```python
from build123d import *

# Parameters (mm, degrees)
SKETCH_1_R           = 20.68
SKETCH_1_R_2         = 9.68
EXTRUDE_1_DEPTH      = 116.68
SKETCH_11_W          = 27
SKETCH_11_H          = 150
CUT_EXTRUDE_3_DEPTH  = 40
SKETCH_13_W          = 10
SKETCH_13_H          = 128.345013401
CUT_EXTRUDE_7_DEPTH  = 126.614916312
SKETCH_15_W          = 8
SKETCH_15_H          = 68.68
CUT_EXTRUDE_9_DEPTH  = 48
SKETCH_16_W          = 15.549431524
SKETCH_16_H          = 20
SKETCH_16_W_2        = 15.459431524
EXTRUDE_4_DEPTH      = 19.2
SKETCH_17_W          = 19.20851187
SKETCH_17_H          = 14.03
CUT_EXTRUDE_10_DEPTH = 20.2
SKETCH_18_R          = 9.59
CUT_EXTRUDE_11_DEPTH = 121.289430957
SKETCH_21_R          = 2.985
CUT_EXTRUDE_12_DEPTH = 55.2
EXTRUDE_START        = 55.2
SKETCH_24_R          = 20.59
SKETCH_24_R_2        = 9.59
EXTRUDE_2_DEPTH      = 55.2
CUT_EXTRUDE_13_DEPTH = 55.2
SKETCH_26_W          = 10.00851187
SKETCH_26_H          = 41.68
CUT_EXTRUDE_15_DEPTH = 55.2
SKETCH_27_W          = 10
SKETCH_27_H          = 40
CUT_EXTRUDE_16_DEPTH = 55.2
SKETCH_28_W          = 44.880694938
SKETCH_28_H          = 9.608044066
CUT_EXTRUDE_17_DEPTH = 12.2
SKETCH_35_W          = 13.53
SKETCH_35_H          = 20
EXTRUDE_10_DEPTH     = 15
EXTRUDE_11_DEPTH     = 15
SKETCH_37_W          = 9
SKETCH_37_H          = 20
EXTRUDE_12_DEPTH     = 20
SKETCH_38_W          = 9
SKETCH_38_H          = 20
EXTRUDE_13_DEPTH     = 20
SKETCH_42_R          = 2.985
CUT_EXTRUDE_21_DEPTH = 20
CUT_EXTRUDE_23_DEPTH = 138.235841092
SKETCH_45_W          = 3
SKETCH_45_H          = 20
EXTRUDE_14_DEPTH     = 30
SKETCH_46_W          = 3
SKETCH_46_H          = 20
EXTRUDE_15_DEPTH     = 30
SKETCH_47_W          = 33.078221107
SKETCH_47_H          = 20
EXTRUDE_16_DEPTH     = 50
SKETCH_48_W          = 30
SKETCH_48_H          = 20
EXTRUDE_17_DEPTH     = 50
SKETCH_50_W          = 50
SKETCH_50_H          = 20
EXTRUDE_18_DEPTH     = 1
SKETCH_51_W          = 50
SKETCH_51_H          = 20
EXTRUDE_19_DEPTH     = 1
SKETCH_52_W          = 53
SKETCH_52_H          = 14
CUT_EXTRUDE_24_DEPTH = 151.972575738
SKETCH_53_W          = 53
SKETCH_53_H          = 14
CUT_EXTRUDE_25_DEPTH = 151.942387436
SKETCH_54_W          = 40
SKETCH_54_H          = 73.27
CUT_EXTRUDE_26_DEPTH = 147.866192927
SKETCH_56_W          = 13.00851187
SKETCH_56_H          = 20
EXTRUDE_21_DEPTH     = 3.08
SKETCH_57_R          = 2.985
CUT_EXTRUDE_27_DEPTH = 127.558817396


with BuildPart() as part:
    # 草圖1 → 伸長-薄件1 (new body)
    with BuildSketch(Plane(origin=(0, 0, 0), x_dir=(1, 0, 0), z_dir=(0, 1, 0))):
        Circle(SKETCH_1_R)
        Circle(SKETCH_1_R_2, mode=Mode.SUBTRACT)
    extrude(amount=EXTRUDE_1_DEPTH)

    # 草圖11 → 除料-伸長3 (cut)
    with BuildSketch(Plane(origin=(0, 116.68, 0), x_dir=(1, 0, 0), z_dir=(0, 1, 0))):
        with Locations((21.70851187, -44.235815192)):
            Rectangle(SKETCH_11_W, SKETCH_11_H)
    extrude(amount=-CUT_EXTRUDE_3_DEPTH, mode=Mode.SUBTRACT)

    # 草圖13 → 除料-伸長7 (cut, through all)
    with BuildSketch(Plane.XY.offset(21)):
        with Locations((-16, 58.612182466)):
            Rectangle(SKETCH_13_W, SKETCH_13_H)
    extrude(amount=-CUT_EXTRUDE_7_DEPTH, mode=Mode.SUBTRACT)

    # 草圖15 → 除料-伸長9 (cut)
    with BuildSketch(Plane.XY.offset(21)):
        with Locations((-1.395744065, 52.34)):
            Rectangle(SKETCH_15_W, SKETCH_15_H)
    extrude(amount=-CUT_EXTRUDE_9_DEPTH, mode=Mode.SUBTRACT)

    # 草圖16 → 填料-伸長4 (add)
    with BuildSketch(Plane(origin=(8.20851187, 0, 0), x_dir=(0, 0, -1), z_dir=(1, 0, 0))):
        with Locations((12.905284238, 106.68)):
            Rectangle(SKETCH_16_W, SKETCH_16_H)
        with Locations((-12.860284238, 106.68)):
            Rectangle(SKETCH_16_W_2, SKETCH_16_H)
    extrude(amount=-EXTRUDE_4_DEPTH)

    # 草圖17 → 除料-伸長10 (cut)
    with BuildSketch(Plane(origin=(0, 116.68, 0), x_dir=(1, 0, 0), z_dir=(0, 1, 0))):
        with Locations((-1.395744065, -0.045)):
            Rectangle(SKETCH_17_W, SKETCH_17_H)
    extrude(amount=-CUT_EXTRUDE_10_DEPTH, mode=Mode.SUBTRACT)

    # 草圖18 → 除料-伸長11 (cut, through all)
    with BuildSketch(Plane.XZ):
        with Locations(Location((0, 0, 0), (0, 0, 90))):
            Circle(SKETCH_18_R)
    extrude(amount=-CUT_EXTRUDE_11_DEPTH, mode=Mode.SUBTRACT)

    # 草圖21 → 除料-伸長12 (cut)
    with BuildSketch(Plane(origin=(0, 0, -20.68), x_dir=(-1, 0, 0), z_dir=(0, 0, -1))):
        with Locations((1.39148813, 108.73)):
            Circle(SKETCH_21_R)
    extrude(amount=-CUT_EXTRUDE_12_DEPTH, mode=Mode.SUBTRACT)

    # 草圖24 → 伸長-薄件2 (add)
    with BuildSketch(Plane.XZ.offset(EXTRUDE_START)):
        Circle(SKETCH_24_R)
        Circle(SKETCH_24_R_2, mode=Mode.SUBTRACT)
    extrude(amount=-EXTRUDE_2_DEPTH)

    # 草圖25 → 除料-伸長13 (cut)
    with BuildSketch(Plane.XY.offset(21)):
        Polygon((-1.39148813, -11.785), (22.612379708, -11.785), (22.612379708, -63.873337429), (-22.749525245, -63.873337429), (-22.749525245, -11.785), align=None)
    extrude(amount=-CUT_EXTRUDE_13_DEPTH, mode=Mode.SUBTRACT)

    # 草圖26 → 除料-伸長15 (cut)
    with BuildSketch(Plane(origin=(0, 0, 0), x_dir=(1, 0, 0), z_dir=(0, 1, 0))):
        with Locations((-15.995744065, -0.16)):
            Rectangle(SKETCH_26_W, SKETCH_26_H)
    extrude(amount=-CUT_EXTRUDE_15_DEPTH, mode=Mode.SUBTRACT)

    # 草圖27 → 除料-伸長16 (cut)
    with BuildSketch(Plane(origin=(21, 0, 0), x_dir=(0, 0, -1), z_dir=(1, 0, 0))):
        with Locations((0, 41.68)):
            Rectangle(SKETCH_27_W, SKETCH_27_H)
    extrude(amount=-CUT_EXTRUDE_16_DEPTH, mode=Mode.SUBTRACT)

    # 草圖28 → 除料-伸長17 (cut)
    with BuildSketch(Plane(origin=(21, 0, 0), x_dir=(0, 0, -1), z_dir=(1, 0, 0))):
        Rectangle(SKETCH_28_W, SKETCH_28_H)
    extrude(amount=-CUT_EXTRUDE_17_DEPTH, mode=Mode.SUBTRACT)

    # 草圖35 → 填料-伸長10 (add)
    with BuildSketch(Plane.ZY.offset(10.99148813)):
        with Locations((13.825, 106.68)):
            Rectangle(SKETCH_35_W, SKETCH_35_H)
    extrude(amount=EXTRUDE_10_DEPTH)

    # 草圖36 → 填料-伸長11 (add)
    with BuildSketch(Plane.ZY.offset(10.99148813)):
        Polygon((-20.68, 116.68), (-6.97, 116.68), (-6.97, 96.48), (-20.68, 96.68), align=None)
    extrude(amount=EXTRUDE_11_DEPTH)

    # 草圖37 → 填料-伸長12 (add)
    with BuildSketch(Plane.XY.offset(20.59)):
        with Locations((-21.49148813, 106.68)):
            Rectangle(SKETCH_37_W, SKETCH_37_H)
    extrude(amount=EXTRUDE_12_DEPTH)

    # 草圖38 → 填料-伸長13 (add)
    with BuildSketch(Plane(origin=(0, 0, -20.68), x_dir=(-1, 0, 0), z_dir=(0, 0, -1))):
        with Locations((21.49148813, 106.68)):
            Rectangle(SKETCH_38_W, SKETCH_38_H)
    extrude(amount=EXTRUDE_13_DEPTH)

    # 草圖42 → 除料-伸長21 (cut)
    with BuildSketch(Plane(origin=(-16.99148813, 0, 0), x_dir=(0, 0, -1), z_dir=(1, 0, 0))):
        with Locations((30.68, 106.554418142)):
            Circle(SKETCH_42_R)
        with Locations((-30.395640125, 106.68)):
            Circle(SKETCH_42_R)
    extrude(amount=-CUT_EXTRUDE_21_DEPTH, mode=Mode.SUBTRACT)

    # 草圖43 → 除料-伸長23 (cut, through all)
    with BuildSketch(Plane(origin=(0, 116.68, 0), x_dir=(1, 0, 0), z_dir=(0, 1, 0))):
        Polygon((-11, 6.97), (-10.99148813, 20.68), (-10.99148813, 48.096794253), (-28.274756234, 48.096794253), (-28.274756234, -43.270506289), (-11, -43.270506289), align=None)
    extrude(amount=-CUT_EXTRUDE_23_DEPTH, mode=Mode.SUBTRACT)

    # 草圖45 → 填料-伸長14 (add)
    with BuildSketch(Plane.XY.offset(20.59)):
        with Locations((-9.5, 106.68)):
            Rectangle(SKETCH_45_W, SKETCH_45_H)
    extrude(amount=EXTRUDE_14_DEPTH)

    # 草圖46 → 填料-伸長15 (add)
    with BuildSketch(Plane(origin=(0, 0, -20.68), x_dir=(-1, 0, 0), z_dir=(0, 0, -1))):
        with Locations((9.49148813, 106.68)):
            Rectangle(SKETCH_46_W, SKETCH_46_H)
    extrude(amount=EXTRUDE_15_DEPTH)

    # 草圖47 → 填料-伸長16 (add)
    with BuildSketch(Plane.ZY.offset(11)):
        with Locations((34.050889447, 106.68)):
            Rectangle(SKETCH_47_W, SKETCH_47_H)
    extrude(amount=EXTRUDE_16_DEPTH)

    # 草圖48 → 填料-伸長17 (add)
    with BuildSketch(Plane.ZY.offset(10.99148813)):
        with Locations((-35.68, 106.68)):
            Rectangle(SKETCH_48_W, SKETCH_48_H)
    extrude(amount=EXTRUDE_17_DEPTH)

    # 草圖50 → 填料-伸長18 (add)
    with BuildSketch(Plane(origin=(0, 0, 17.511778893), x_dir=(-1, 0, 0), z_dir=(0, 0, -1))):
        with Locations((36, 106.68)):
            Rectangle(SKETCH_50_W, SKETCH_50_H)
    extrude(amount=EXTRUDE_18_DEPTH)

    # 草圖51 → 填料-伸長19 (add)
    with BuildSketch(Plane.XY.offset(-20.68)):
        with Locations((-35.99148813, 106.68)):
            Rectangle(SKETCH_51_W, SKETCH_51_H)
    extrude(amount=EXTRUDE_19_DEPTH)

    # 草圖52 → 除料-伸長24 (cut, through all)
    with BuildSketch(Plane(origin=(0, 116.68, 0), x_dir=(1, 0, 0), z_dir=(0, 1, 0))):
        with Locations((-34.49148813, 43.68)):
            Rectangle(SKETCH_52_W, SKETCH_52_H)
    extrude(amount=-CUT_EXTRUDE_24_DEPTH, mode=Mode.SUBTRACT)

    # 草圖53 → 除料-伸長25 (cut, through all)
    with BuildSketch(Plane(origin=(0, 116.68, 0), x_dir=(1, 0, 0), z_dir=(0, 1, 0))):
        with Locations((-34.5, -43.59)):
            Rectangle(SKETCH_53_W, SKETCH_53_H)
    extrude(amount=-CUT_EXTRUDE_25_DEPTH, mode=Mode.SUBTRACT)

    # 草圖54 → 除料-伸長26 (cut, through all)
    with BuildSketch(Plane(origin=(0, 116.68, 0), x_dir=(1, 0, 0), z_dir=(0, 1, 0))):
        with Locations((-41, 0.045)):
            Rectangle(SKETCH_54_W, SKETCH_54_H)
    extrude(amount=-CUT_EXTRUDE_26_DEPTH, mode=Mode.SUBTRACT)

    # 草圖56 → 填料-伸長21 (add)
    with BuildSketch(Plane(origin=(0, 0, -36.68), x_dir=(-1, 0, 0), z_dir=(0, 0, -1))):
        with Locations((14.495744065, 106.68)):
            Rectangle(SKETCH_56_W, SKETCH_56_H)
    extrude(amount=EXTRUDE_21_DEPTH)

    # 草圖57 → 除料-伸長27 (cut, through all)
    with BuildSketch(Plane(origin=(-7.99148813, 0, 0), x_dir=(0, 0, -1), z_dir=(1, 0, 0))):
        with Locations((30.22, 106.634392252)):
            Circle(SKETCH_57_R)
        with Locations((-28.59, 106.68)):
            Circle(SKETCH_57_R)
    extrude(amount=-CUT_EXTRUDE_27_DEPTH, mode=Mode.SUBTRACT)


solid = part.part
```
Geometry check sheet. Reference: the model listing, model coordinates, mm. A direction names the side the tool comes from. Coordinates: 2 decimals unless noted, no trailing zeros. Loops run counter-clockwise (first coordinate to the right, second up) from the corner with the lowest first, then second, coordinate; pieces in that order, holes last. Notation, with made-up numbers: (28.25, -28.5) - (82.25, -28.5) arc R24 ccw to (82.25, 0.5) - close; hole circle Ø10 at (-3, -8). An arc over 180 degrees is marked (long way). One line per item, written item: value. Start each with the question number.
(1) Depth check by flat-ended pin: P1, Ø6, axis at x = -7, y = 71.5, coming from the -Z side; P2, Ø6, axis at y = 37.5, z = -14, coming from the +X side; P3, Ø2, axis at y = 9.5, z = 9.5, coming from the +X side. Enter the tip coordinate at first touch or a pass-through.
(2) Cross-section at C-C on x = 17.5. Enter the section's corners in (y, z) (3 decimals), plus the area to 3 significant figures.
(3) Cross-section at B-B on y = 69.5. Enter the section's corners in (x, z), plus the area to 3 significant figures.
(4) Tool access check on faces 4 (the cylindrical face through (18.678, 44.559, -8.876)), 5 (the flat face through (-1, 18, -14)), 6 (the flat face through (-9, 107, -6.97)), 7 (the flat face through (-10, 61.68, 0)). Record the directions out of +Z, -Z, +X, -X, +Y, -Y that give a thin tool (end or side, any length) a straight path to the whole face; none if there is none.
(5) Mould release check, pull along Y, two halves, no side actions. Record for faces 1 (the flat face through (-8, 107, 25)), 2 (the flat face through (13, -4.804, 0)), 3 (the flat face through (-13, 96.68, 27)): released by +Y, released by -Y, zero draft, split by the parting line, or undercut.
(6) Material ranges on line 1 (Y direction, x = 10.5, z = -0.5) (3 decimals); line 2 (Y direction, x = 9, z = 10.5) (3 decimals); line 3 (X direction, y = 78.5, z = -11.5), recorded low to high. Write a range as [from, to].
(7) Cross-section at A-A on z = 0. Enter the section's corners in (x, y) (3 decimals), plus the area to 3 significant figures.
(8) Cross-section at D-D on z = -30.22. Enter the section's corners in (x, y), plus the area to 3 significant figures.
Results below:
1. P1: stops at z = -19.96
1. P2: stops at x = 17.51
1. P3: stops at x = 18.85
2. outline: (-11.785, -10.849) - (-4.804, -10.849) - (-4.804, 10.849) - (-11.785, 10.849) - close; (4.804, -11.019) - (76.68, -11.019) - (76.68, 11.019) - (4.804, 11.019) - close; hole (21.68, -5) - (61.68, -5) - (61.68, 5) - (21.68, 5) - close
2. area: 1,340 mm2
3. outline: (-11, -6.97) - (-10.99, -17.52) arc R20.68 ccw to (-5.4, -19.96) - (-5.4, -8.04) arc R9.68 cw to (-5.4, 8.04) - (-5.4, 19.96) arc R20.68 ccw to (-11, 17.51) - close; (2.6, -20.52) arc R20.68 ccw to (2.6, 20.52) - (2.6, 9.32) arc R9.68 cw to (2.6, -9.32) - close
3. area: 630 mm2
4. face 4: -Y
4. face 5: +Z, -Z
4. face 6: +X, -X, +Y
4. face 7: +X, -X
5. face 1: zero draft
5. face 2: undercut
5. face 3: released by -Y
6. line 1: y = [-11.785, -4.804], [4.804, 21.68], [61.68, 76.68]
6. line 2: y = [-11.785, -4.804], [4.804, 76.68]
6. line 3: x = [-11, -5.4], [2.6, 8.21]
7. outline: (-11, 0) - (-10.991, 0) - (-10.991, -11.785) - (-9.59, -11.785) - (-9.59, 0) - (-9.68, 0) - (-9.68, 21.68) - (-11, 21.68) - close; (-11, 61.68) - (-9.68, 61.68) - (-9.68, 96.48) - (-11, 96.48) - close; (9.59, -11.785) - (20.59, -11.785) - (20.59, -4.804) - (9.59, -4.804) - close; (9.68, 4.804) - (20.68, 4.804) - (20.68, 21.68) - (9.68, 21.68) - close; (9.68, 61.68) - (20.68, 61.68) - (20.68, 76.68) - (9.68, 76.68) - close
7. area: 518 mm2
8. outline: (-21, 96.68) - (-7.99, 96.68) - (-7.99, 103.65) - (-21, 103.65) - close; (-21, 109.62) - (-7.99, 109.62) - (-7.99, 116.68) - (-21, 116.68) - close
8. area: 183 mm2
